```python
from build123d import *

# Parameters (mm, degrees)
SHELL1_T               = -2
BOSS_EXTRUDE1_START    = 2
SKETCH7_6_W            = 6
SKETCH7_6_H            = 2
BOSS_EXTRUDE1_DEPTH    = 33.5
SKETCH7_9_W            = 2
SKETCH7_9_H            = 1.4
SKETCH7_9_W_2          = 2.3
SKETCH7_9_W_3          = 0.6
BOSS_EXTRUDE3_DEPTH    = 35.5
SKETCH7_8_W            = 1.6
SKETCH7_8_H            = 1.4
SKETCH7_8_W_2          = 1.3
SKETCH7_8_W_3          = 0.3
BOSS_EXTRUDE2_DEPTH    = 63.8
FILLET1_R              = 1.4
CUT_EXTRUDE1_START     = -46.163243618
CUT_EXTRUDE1_OUTLINE_W = 62.3
CUT_EXTRUDE1_OUTLINE_H = 22.2
CUT_EXTRUDE1_DEPTH     = 6.326424063
CUT_EXTRUDE2_START     = -2
SKETCH11_R             = 2.5
CUT_EXTRUDE2_DEPTH     = 96


# Read off the part's stored shape, not the designer's step: Cut-Extrude1
with BuildPart() as part:
    # Sketch7 → Loft1 section 0
    with BuildSketch(Plane(origin=(0, 0, 0), x_dir=(1, 0, 0), z_dir=(0, 1, 0))):
        with BuildLine():
            Line((0, 96), (35.41423357, 96))
            ThreePointArc((35.41423357, 96), (43.772922591, 48), (35.41423357, 0))
            Line((35.41423357, 0), (0, 0))
            Line((0, 0), (0, 96))
        make_face()
    # Sketch9 → Loft1 section 1
    with BuildSketch(Plane(origin=(0, 66, 0), x_dir=(1, 0, 0), z_dir=(0, 1, 0))):
        with BuildLine():
            Line((0, 96), (38.124209432, 96))
            ThreePointArc((38.124209432, 96), (46.317469671, 48), (38.124209432, 0))
            Line((38.124209432, 0), (0, 0))
            Line((0, 0), (0, 96))
        make_face()
    loft()

    # Shell1
    shell1_openings = [part.faces().sort_by_distance(p)[0] for p in [
        (21.876860879, 66, -48),
    ]]
    offset(amount=SHELL1_T, openings=shell1_openings, kind=Kind.INTERSECTION)

    # Sketch7<6> → Boss-Extrude1 (add)
    with BuildSketch(Plane(origin=(0, 0, 0), x_dir=(1, 0, 0), z_dir=(0, 1, 0)).offset(BOSS_EXTRUDE1_START)):
        with Locations((5, 31.6)):
            Rectangle(SKETCH7_6_W, SKETCH7_6_H)
        Polygon((18, 32.6), (18, 30.6), (26, 30.6), (26, 94), (24, 94), (24, 32.6), align=None)
    extrude(amount=BOSS_EXTRUDE1_DEPTH)

    # Sketch7<9> → Boss-Extrude3 (add)
    with BuildSketch(Plane(origin=(0, 0, 0), x_dir=(1, 0, 0), z_dir=(0, 1, 0))):
        with Locations((3, 2.7)):
            Rectangle(SKETCH7_9_W, SKETCH7_9_H)
        with Locations((25.45, 2.7)):
            Rectangle(SKETCH7_9_W_2, SKETCH7_9_H)
        with Locations((3, 93.3)):
            Rectangle(SKETCH7_9_W, SKETCH7_9_H)
        with Locations((26.3, 93.3)):
            Rectangle(SKETCH7_9_W_3, SKETCH7_9_H)
    extrude(amount=BOSS_EXTRUDE3_DEPTH)

    # Sketch7<8> → Boss-Extrude2 (add)
    with BuildSketch(Plane(origin=(0, 0, 0), x_dir=(1, 0, 0), z_dir=(0, 1, 0))):
        with Locations((4.8, 2.7)):
            Rectangle(SKETCH7_8_W, SKETCH7_8_H)
        with Locations((27.4, 2.7)):
            Rectangle(SKETCH7_8_W, SKETCH7_8_H)
        with Locations((23.5, 2.7)):
            Rectangle(SKETCH7_8_W, SKETCH7_8_H)
        with Locations((4.8, 93.3)):
            Rectangle(SKETCH7_8_W, SKETCH7_8_H)
        with Locations((27.4, 93.3)):
            Rectangle(SKETCH7_8_W, SKETCH7_8_H)
        with Locations((23.35, 93.3)):
            Rectangle(SKETCH7_8_W_2, SKETCH7_8_H)
        with Locations((24.15, 93.3)):
            Rectangle(SKETCH7_8_W_3, SKETCH7_8_H)
    extrude(amount=BOSS_EXTRUDE2_DEPTH)

    # Fillet1
    fillet1_edges = [part.edges().sort_by_distance(p)[0] for p in [
        (22.7, 32.9, -94),
        (28.2, 32.9, -94),
        (5.6, 32.9, -94),
        (2, 18.75, -32.6),
        (2, 18.75, -30.6),
        (5.6, 32.9, -2),
        (22.7, 32.9, -2),
        (28.2, 32.9, -2),
    ]]
    fillet(fillet1_edges, radius=FILLET1_R - 0.0001)  # a hair under: the kernel refuses the full size

    # Cut-Extrude1 outline → Cut-Extrude1 (cut)
    with BuildSketch(Plane.ZY.offset(CUT_EXTRUDE1_START)):
        with Locations((-48, 50.9)):
            Rectangle(CUT_EXTRUDE1_OUTLINE_W, CUT_EXTRUDE1_OUTLINE_H)
    extrude(amount=CUT_EXTRUDE1_DEPTH, mode=Mode.SUBTRACT)

    # Sketch11 → Cut-Extrude2 (cut)
    with BuildSketch(Plane.XY.offset(-94).offset(CUT_EXTRUDE2_START)):
        with Locations(Location((31.825322124, 32.5, 0), (0, 0, 180))):
            Circle(SKETCH11_R)
    extrude(amount=CUT_EXTRUDE2_DEPTH, mode=Mode.SUBTRACT)


solid = part.part
```
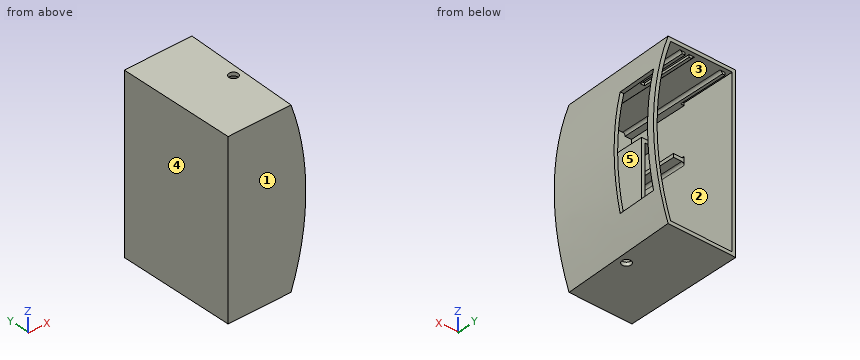
The model under review builds one solid part; all positions refer to its coordinate system, in mm. Face numbers are marked on the shaded views. A direction names the side the tool comes from. Round coordinates to 2 decimals unless told otherwise and drop trailing zeros. Use a Markdown table: item, result.
1) Consider section A-A (x = 32.5). Give the number of separate pieces and of enclosed holes in the cut face, then the cut area to 3 significant figures.
Report:
| item | result |
|---|---|
| separate pieces | 3 |
| enclosed holes | 0 |
| area | 429 mm^2 |
2) Insertion check: pin 1 (3 mm diameter, centred on x = 5.5, z = -47.5, fed in from +Y); pin 2 (10 mm diameter, centred on y = 14, z = -59.5, fed in from +X); pin 3 (12 mm diameter, centred on x = 27.5, z = -62.5, fed in from +Y); pin 4 (3 mm diameter, centred on x = 31.83, y = 32.5, fed in from -Z). Each pin has a flat end and moves straight along its axis. Give the tip position at first contact, or say it passes through.
Report:
| item | result |
|---|---|
| pin 1 | y = 2 |
| pin 2 | x = 44.23 |
| pin 3 | y = 35.5 |
| pin 4 | through |
3) Wall thickness on line 1 along X through (y, z) = (32, -84); line 2 along Z through (x, y) = (11, 43.5); line 3 along X through (y, z) = (11, -60): over which ranges is each line inside the solid? List them lowest first. Write a range as [from, to].
Report:
| item | result |
|---|---|
| line 1 | [0, 2], [24, 26], [38.34, 40.41] |
| line 2 | [-96, -94], [-2, 0] |
| line 3 | [0, 2], [24, 26], [41.68, 43.69] |
4) Draft analysis for pull direction Z (two halves, no side actions). For the marked faces 1, 2 and 3, state which applies: released by +Z, released by -Z, zero draft, split by the parting line, or undercut.
Report:
| item | result |
|---|---|
| face 1 | zero draft |
| face 2 | undercut |
| face 3 | undercut |
5) Tool access review of the marked faces 4 and 5: name each direction out of +Z, -Z, +X, -X, +Y, -Y from which nothing blocks a thin tool from reaching the whole face with its end or side.
Report:
| item | result |
|---|---|
| face 4 | +Z, -Z, -X, +Y, -Y |
| face 5 | +Y |
